Can you work these out from the model? Positions are in its coordinate system, mm. Face numbers are marked on the shaded views. A direction names the side the tool comes from. Round coordinates to 2 decimals unless told otherwise and drop trailing zeros. Write each loop counter-clockwise with the first axis right and the second up, starting at its lowest first coordinate (ties: lowest second). Pieces come first, ordered by that corner, then holes.
Q1. I'm going to push flat-ended pins straight in: pin 1 Ø5 at (x, y) = (-9.5, 36.5) entering from -Z; pin 2 Ø2 at (y, z) = (93.5, 8) entering from +X; pin 3 Ø3 at (y, z) = (65, 3.5) entering from -X. Where does each tip first touch, or does it pass through?
Q2. If we section it at B-B (x = 0): Please give me the cut outline in (y, z).
Q3. For the marked faces 1 and 2, which set-ups out of +Z, -Z, +X, -X, +Y, -Y let a thin tool reach every point of the face, with its end or its side?
Q4. Please list where these lines run through material, in increasing order: line 1 along Z through (x, y) = (-0.25, 7); line 2 along Y through (x, z) = (-1, 11.25); line 3 along X through (y, z) = (12, -1).
Q5. If we section it at C-C (y = 34.5): Please give me the cut outline in (x, z).
Q6. We'd pull the mould along X, two halves only. Please class the marked faces 3, 4 and 5: +X half, -X half, draft (parallel to the pull), parting line (faces both ways), or undercut.
Q7. If we section it at A-A (z = 0): Please give me the cut outline in (x, y), plus the area to 3 significant figures.
from build123d import *

# Parameters (mm, degrees)
CHAMFER1_SIZE     = 1
M8_TAPPED_HOLE1_D = 6.8


with BuildPart() as part:
    # Sketch1 → Revolve1 (revolve)
    with BuildSketch(Plane(origin=(0, 0, 0), x_dir=(0, 0, -1), z_dir=(1, 0, 0))):
        Polygon((0, 0), (0, 127), (-10, 127), (-10, 52), (-12, 52), (-12, 50), (-9.95, 50), (-9.95, 0), align=None)
    revolve(axis=Axis((0, 0, 0), (0, 1, 0)))

    # Chamfer1
    chamfer1_edges = [part.edges().sort_by_distance(p)[0] for p in [
        (0, 0, -9.95),
        (0, 127, -10),
    ]]
    chamfer(chamfer1_edges, length=CHAMFER1_SIZE)

    # M8 Tapped Hole1 (through all)
    with Locations(Plane(origin=(0, 127, 0), x_dir=(1, 0, 0), z_dir=(0, 1, 0))):
        with Locations((0, 0)):
            Hole(M8_TAPPED_HOLE1_D / 2)


solid = part.part
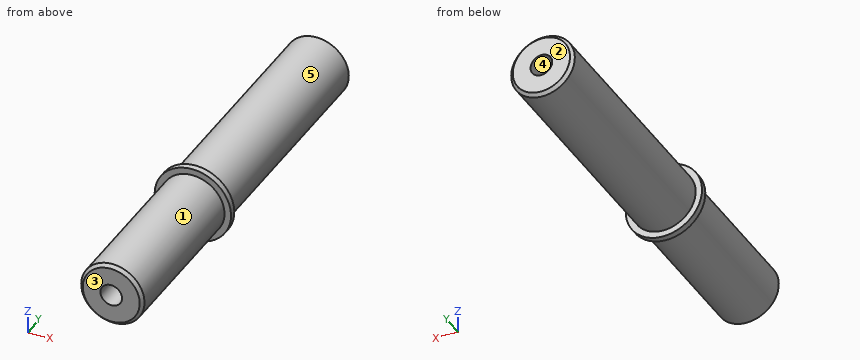
A:
1. pin 1: stops at z = -7.07
1. pin 2: stops at x = 7.14
1. pin 3: stops at x = -9.8
2. outline: (0, -8.95) - (1, -9.95) - (50, -9.95) - (50, -12) - (52, -12) - (52, -10) - (126, -10) - (127, -9) - (127, -3.4) - (0, -3.4) - close; (0, 3.4) - (127, 3.4) - (127, 9) - (126, 10) - (52, 10) - (52, 12) - (50, 12) - (50, 9.95) - (1, 9.95) - (0, 8.95) - close
3. face 1: -Y
3. face 2: +Z, -Z, +X, -X, +Y
4. line 1: z = -9.95 to -3.39, 3.39 to 9.95
4. line 2: y = 50 to 52
4. line 3: x = -9.9 to -3.25, 3.25 to 9.9
5. outline: circle Ø19.9 at (0, 0); hole circle Ø6.8 at (0, 0)
6. face 3: draft
6. face 4: undercut
6. face 5: parting line
7. outline: (-12, 50) - (-9.95, 50) - (-9.95, 1) - (-8.95, 0) - (-3.4, 0) - (-3.4, 127) - (-9, 127) - (-10, 126) - (-10, 52) - (-12, 52) - close; (3.4, 0) - (8.95, 0) - (9.95, 1) - (9.95, 50) - (12, 50) - (12, 52) - (10, 52) - (10, 126) - (9, 127) - (3.4, 127) - close
7. area: 1,680 mm2
